Geometry check sheet. Reference: the model listing, model coordinates, mm. Face numbers are marked on the shaded views. A direction names the side the tool comes from. Give positions to 0.01 mm unless a question says otherwise; leave off trailing zeros. Order: outer loops, then holes, each group sorted by start corner. A loop starts at its lowest first (then second) coordinate and runs counter-clockwise, first axis right, second up. Notation, with made-up numbers: M 66,-32.75 L 120,-32.75 A31 cw 120,3.25 Z; hole C 34,29.5 d1. An arc over 180 degrees is marked long. Answer as a JSON object with one key per item and string values. Group by question number.
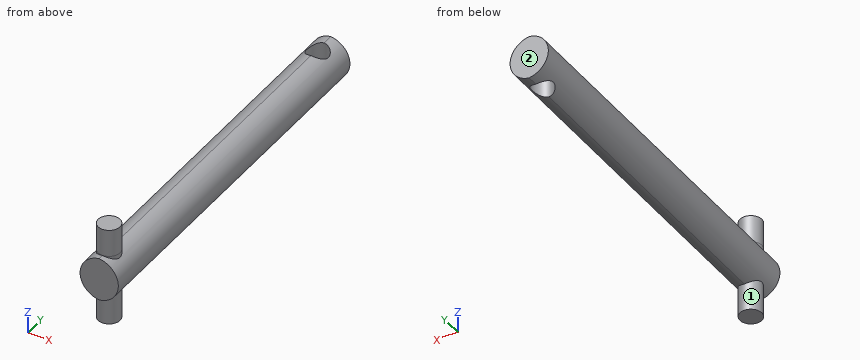
from build123d import *

# Parameters (mm, degrees)
SKETCH2_W           = 7
SKETCH2_H           = 8
BOSS_EXTRUDE1_DEPTH = 70
SKETCH3_R           = 2
BOSS_EXTRUDE2_DEPTH = 5
CUT_EXTRUDE1_REACH  = 73.283
SKETCH4_R           = 2
FILLET1_R           = 4


with BuildPart() as part:
    # Sketch2 → Boss-Extrude1 (new body)
    with BuildSketch(Plane(origin=(0, 0, 0), x_dir=(1, 0, 0), z_dir=(0, 1, 0))):
        Rectangle(SKETCH2_W, SKETCH2_H)
    extrude(amount=BOSS_EXTRUDE1_DEPTH)

    # Sketch3 → Boss-Extrude2 (add)
    with BuildSketch(Plane.XY.offset(4)):
        with Locations(Location((0, 3, 0), (0, 0, 180))):
            Circle(SKETCH3_R)
    boss_extrude2 = extrude(amount=BOSS_EXTRUDE2_DEPTH)

    # Mirror1: Boss-Extrude2 across plane
    add(boss_extrude2.mirror(Plane.XY))

    # Sketch4 → Cut-Extrude1 (cut, up to next)
    with BuildSketch(Plane.XY.offset(4), mode=Mode.PRIVATE) as cut_extrude1_sk1:
        with Locations((0, 66)):
            Circle(SKETCH4_R)
    cut_extrude1_tool1 = extrude(cut_extrude1_sk1.sketch, amount=-CUT_EXTRUDE1_REACH, mode=Mode.PRIVATE) & part.part
    add(cut_extrude1_tool1.solids().sort_by_distance((0, 66, 4))[0], mode=Mode.SUBTRACT)

    # Fillet1
    # the kernel refuses this fillet: 4 mm, written as the material it takes off along each edge
    with BuildSketch(Plane(origin=(-3.5, -10, 4), x_dir=(0, 0, -1), z_dir=(0, 1, 0))) as fillet1_piece_1_section:
        with BuildLine():
            CenterArc((FILLET1_R, -FILLET1_R), FILLET1_R, 90, 90)
            Line((0, -FILLET1_R), (0, 0))
            Line((0, 0), (FILLET1_R, 0))
        make_face()
    fillet1_piece_1 = extrude(amount=90, mode=Mode.PRIVATE)
    fillet1_piece_1 = fillet1_piece_1 - Plane(origin=(0, 3, 3.08936477), x_dir=(-1, 0, 0), z_dir=(0, 0, -1)) * Cylinder(2, 196, mode=Mode.PRIVATE)
    add(fillet1_piece_1, mode=Mode.SUBTRACT)
    with BuildSketch(Plane(origin=(-3.5, -10, -4), x_dir=(1, 0, 0), z_dir=(0, 1, 0))) as fillet1_piece_2_section:
        with BuildLine():
            CenterArc((FILLET1_R, -FILLET1_R), FILLET1_R, 90, 90)
            Line((0, -FILLET1_R), (0, 0))
            Line((0, 0), (FILLET1_R, 0))
        make_face()
    fillet1_piece_2 = extrude(amount=90, mode=Mode.PRIVATE)
    fillet1_piece_2 = fillet1_piece_2 - Plane(origin=(0, 3, -3.089364757), x_dir=(-1, 0, 0), z_dir=(0, 0, 1)) * Cylinder(2, 196, mode=Mode.PRIVATE)
    add(fillet1_piece_2, mode=Mode.SUBTRACT)
    with BuildSketch(Plane(origin=(3.5, -10, -4), x_dir=(-1, 0, 0), z_dir=(0, 1, 0))) as fillet1_piece_3_section:
        with BuildLine():
            CenterArc((FILLET1_R, FILLET1_R), FILLET1_R, 180, 90)
            Line((0, FILLET1_R), (0, 0))
            Line((0, 0), (FILLET1_R, 0))
        make_face()
    fillet1_piece_3 = extrude(amount=90, mode=Mode.PRIVATE)
    fillet1_piece_3 = fillet1_piece_3 - Plane(origin=(0, 3, -3.089364802), x_dir=(-1, 0, 0), z_dir=(0, 0, 1)) * Cylinder(2, 196, mode=Mode.PRIVATE)
    add(fillet1_piece_3, mode=Mode.SUBTRACT)
    with BuildSketch(Plane(origin=(3.5, -10, 4), x_dir=(0, 0, -1), z_dir=(0, 1, 0))) as fillet1_piece_4_section:
        with BuildLine():
            CenterArc((FILLET1_R, FILLET1_R), FILLET1_R, 180, 90)
            Line((0, FILLET1_R), (0, 0))
            Line((0, 0), (FILLET1_R, 0))
        make_face()
    fillet1_piece_4 = extrude(amount=90, mode=Mode.PRIVATE)
    fillet1_piece_4 = fillet1_piece_4 - Plane(origin=(0, 3, 3.089364961), x_dir=(-1, 0, 0), z_dir=(0, 0, -1)) * Cylinder(2, 196, mode=Mode.PRIVATE)
    add(fillet1_piece_4, mode=Mode.SUBTRACT)


solid = part.part
1. Access from +Z, -Z, +X, -X, +Y, -Y to the whole of each face (thin tool, end or side, straight path). Record for the marked faces 1 and 2.
2. Thickness scan on line 1 along Y through (x, z) = (0, 0.5); line 2 along X through (y, z) = (66, 2.75); line 3 along X through (y, z) = (66, -0.5). Record the ranges inside material, lowest first. Write a range as [from, to].
3. Cross-section at C-C (y = 38). Record the cut outline in (x, z).
4. Cross-section at A-A (y = 3). Record the cut outline in (x, z), and give its area (3 significant figures).
5. Depth check by flat-ended pin: pin 1 (2.5 mm diameter, centred on x = 0, y = 66, fed in from -Z); pin 2 (1.5 mm diameter, centred on y = 33, z = -3, fed in from -X); pin 3 (1.5 mm diameter, centred on x = 1, y = 43.5, fed in from +Z); pin 4 (1.5 mm diameter, centred on x = 1.5, y = 41, fed in from +Z). Enter the tip coordinate at first touch or a pass-through.
6. Cross-section at B-B (y = 66). Record the cut outline in (x, z), and give its area (3 significant figures).
Report:
{
 "1": {"face 1": "-Z", "face 2": "+Z, -Z, +X, -X, +Y"},
 "2": {"line 1": "y = [0, 64], [68, 70]", "line 2": "x = [-2.4, -2], [2, 2.4]", "line 3": "x = [-3.47, -2], [2, 3.47]"},
 "3": {"outline": "M 0,-3.97 A4 ccw 0,3.97 A4 ccw Z"},
 "4": {"outline": "M -2,-9 L 2,-9 L 2,-3.12 A4 ccw 2,3.12 L 2,9 L -2,9 L -2,3.12 A4 ccw -2,-3.12 Z", "area": "85.0 mm2"},
 "5": {"pin 1": "passes through", "pin 2": "stops at x = -2.81", "pin 3": "stops at z = 3.93", "pin 4": "stops at z = 3.8"},
 "6": {"outline": "M -2,-3.12 L -2,3.12 A4 ccw Z; M 2,-3.12 A4 ccw 2,3.12 Z", "area": "13.0 mm2"}
}
